Work out the finished part from the listing and answer in its coordinate system (mm). Face numbers are marked on the shaded views. A direction names the side the tool comes from. Coordinates: 2 decimals unless noted, no trailing zeros. Order: outer loops, then holes, each group sorted by start corner. A loop starts at its lowest first (then second) coordinate and runs counter-clockwise, first axis right, second up.
1. The part is cut by section C-C, the plane y = -16. Give the vertices of the cut face in (x, z), then the cut area to 3 significant figures.
2. Flat-ended cylindrical pins translate along their axes: pin 1 Ø4 at (y, z) = (-20.5, 39.5) entering from -X; pin 2 Ø2 at (x, z) = (-16.5, 40.5) entering from -Y; pin 3 Ø5 at (x, y) = (5, -12) entering from +Z; pin 4 Ø2.5 at (x, y) = (6.96, -25.93) entering from -Z. Find the tip coordinate at first contact, or state that the pin passes through.
3. Find the intervals of material crossed by probe 1 along Y at (x, z) = (-11.5, 23); probe 2 along Z at (x, y) = (-24, -26); probe 3 along X at (y, z) = (-19, 27), in increasing order.
4. The part is cut by section A-A, the plane x = -14.5. Give the vertices of the cut face in (y, z).
5. Determine the mould class of the marked faces 6, 7, 8 and 9 for opening direction Z: +Z half, -Z half, draft (parallel to the pull), parting line (faces both ways), or undercut.
6. The part is cut by section D-D, the plane x = -22. Give the vertices of the cut face in (y, z), then the cut area to 3 significant figures.
7. The part is cut by section B-B, the plane z = 50. Give the vertices of the cut face in (x, y), then the cut area to 3 significant figures.
8. A tool of negligible diameter and unlimited length cuts with its end or side. For the marked faces 1, 2, 3, 4 and 5, from which of +Z, -Z, +X, -X, +Y, -Y can it reach the whole face along a straight path? Write none if from no direction.
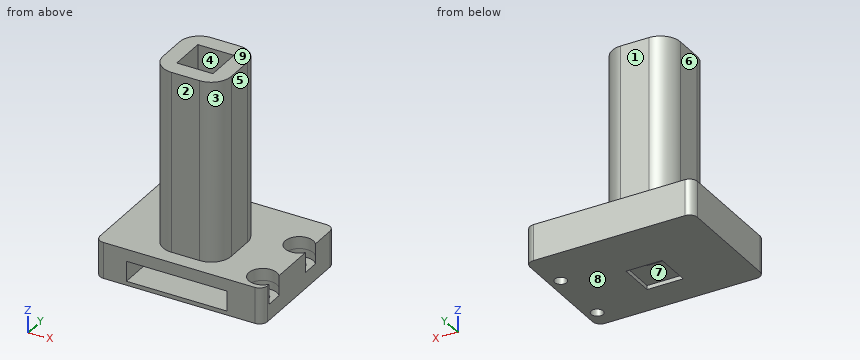
Autodesk Inventor part; units mm, degrees
ref_plane "YZ Plane" through (0, 0, 0) normal (1, 0, 0) x (0, 1, 0)
ref_plane "XZ Plane" through (0, 0, 0) normal (0, 1, 0) x (-1, 0, 0)
ref_plane "XY Plane" through (0, 0, 0) normal (0, 0, 1) x (1, 0, 0)
ref_plane "Work Plane1" through (0, 0, 0) normal (0, 0, 1) x (1, 0, 0)
sketch "Sketch1" plane through (0, 0, 0) normal (0, 0, 1) x (1, 0, 0)
  line L0 (9.7547, 0) -> (-32, 0) construction
  line L1 (-32, 0) -> (-32, -5) construction
  line L2 (-5, -5) -> (-32, -5) construction
  line L3 (-5, -30.7015) -> (-5, -5) construction
  line L4 (-0.2453, -30.7015) -> (-5, -30.7015) construction
  line L5 (-0.2453, -30.7015) -> (-0.2453, -31) construction
  line L6 (-0.2453, -31) -> (4.1607, -31) construction
  line L7 (4.1607, -66) -> (4.1607, -31)
  line L8 (9.7547, -66) -> (4.1607, -66)
  line L9 (9.7547, 0) -> (9.7547, -66)
  circle A0 centre (-2.5, -10.3442) radius 1.45 construction
  circle A1 centre (-2.5, -25.9266) radius 1.45 construction
  circle A2 centre (-11.7453, -18.3978) radius 6 construction
  line L10 (-7.2453, -22.8978) -> (-16.2453, -22.8978)
  line L11 (-16.2453, -22.8978) -> (-16.2453, -13.8978)
  line L12 (-16.2453, -13.8978) -> (-7.2453, -13.8978)
  line L13 (-7.2453, -13.8978) -> (-7.2453, -22.8978)
  line L14 (-7.2453, -22.8978) -> (-16.2453, -13.8978)
  line L15 (-16.2453, -22.8978) -> (-7.2453, -13.8978)
  line L16 (9.7547, 0) -> (-32, 0)
  line L17 (9.7547, 0) -> (-32, 0) construction
  line L18 (-32, 0) -> (-32, -5) construction
  line L19 (-5, -5) -> (-32, -5) construction
  line L20 (-5, -30.7015) -> (-5, -5) construction
  line L21 (-0.2453, -30.7015) -> (-5, -30.7015) construction
  line L22 (-0.2453, -30.7015) -> (-0.2453, -31) construction
  line L23 (-0.2453, -31) -> (4.1607, -31) construction
  line L24 (4.1607, -66) -> (4.1607, -31) construction
  line L25 (9.7547, -66) -> (4.1607, -66) construction
  line L26 (9.7547, 0) -> (9.7547, -66) construction
  circle A3 centre (-2.5, -10.3442) radius 1.45 construction
  circle A4 centre (-2.5, -25.9266) radius 1.45 construction
  line L27 (9.7547, 0) -> (-32, 0)
  line L28 (-32, 0) -> (-32, -30.7015)
  line L29 (-32, -30.7015) -> (9.7547, -30.7015)
  line L30 (9.7547, -30.7015) -> (9.7547, 0)
  circle A5 centre (-2.5, -25.9266) radius 1.65
  circle A6 centre (-2.5, -10.3442) radius 1.65
  circle A7 centre (6.9577, -25.9266) radius 1.45
  circle A8 centre (6.9577, -10.3442) radius 1.45
  circle A9 centre (6.9577, -25.9266) radius 1.45
  circle A10 centre (6.9577, -10.3442) radius 1.45
  point P0 (0, 0)
  dimension "d0" = 9
  dimension "d1" = 9
  dimension "d2" = 3.3
  dimension "d3" = 3.3
extrude "Extrusion1" add sketch "Sketch1" along normal blind 6 contours L9 L29 L28 L16 | A5 | A6 | A7 | A8
sketch "Sketch2" plane through (0, 0, 6) normal (0, 0, 1) x (1, 0, 0)
  circle A0 centre (-2.5, -25.9266) radius 1.65
  circle A1 centre (-2.5, -10.3442) radius 1.65
  circle A2 centre (6.9577, -25.9266) radius 1.45
  circle A3 centre (6.9577, -10.3442) radius 1.45
  point P0 (0, 0)
hole "Hole1" at (6.9577, -25.9266, 6) at (6.9577, -10.3442, 6) direction (0, 0, -1) diameter 3 end through all counterbore diameter 7 counterbore depth 2
fillet "Fillet1" radius 2 4 edges at (-32, 0, 3) (9.7547, 0, 3) (9.7547, -30.7015, 3) (-32, -30.7015, 3)
sketch "Sketch3" plane through (0, 0, 6) normal (0, 0, 1) x (1, 0, 0)
  line L0 (-16.2453, -22.8978) -> (-16.2453, -13.8978)
  line L1 (-7.2453, -13.8978) -> (-7.2453, -22.8978)
  line L2 (-7.2453, -22.8978) -> (-16.2453, -22.8978)
  circle A0 centre (-11.7453, -18.3978) radius 6
  circle A1 centre (-11.7453, -18.3978) radius 12.75
  line L3 (-24.4953, -18.3978) -> (1.0047, -18.3978)
  line L4 (0.7547, -46.1354) -> (-24.2453, -46.1354)
  line L5 (-24.2453, -46.1354) -> (-24.2453, -20.9102)
  line L6 (-24.2453, -20.9102) -> (0.7547, -20.9102)
  line L7 (0.7547, -20.9102) -> (0.7547, -46.1354)
  line L8 (0.7547, -46.1354) -> (-24.2453, -20.9102) construction
  line L9 (-24.2453, -46.1354) -> (0.7547, -20.9102) construction
  point P0 (0, 0)
  point P1 (-11.7453, -33.5228)
  dimension "d14" = 25.5
  dimension "d17" = 25
extrude "Extrusion2" cut sketch "Sketch3" against normal blind 5
sketch "Sketch4" plane through (0, 0, 6) normal (0, 0, 1) x (1, 0, 0)
  line L0 (0.7547, -20.9102) -> (0.7547, -30.7015)
  line L1 (0.7547, -30.7015) -> (7.7547, -30.7015)
  arc A0 (7.7547, -30.7015) -> (9.7547, -28.7015) centre (7.7547, -28.7015) ccw
  line L2 (9.7547, -28.7015) -> (9.7547, -28.0305)
  arc A1 (9.7547, -23.8226) -> (9.7547, -28.0305) centre (6.9577, -25.9266) ccw
  line L3 (9.7547, -23.8226) -> (9.7547, -12.4481)
  arc A2 (9.7547, -8.2402) -> (9.7547, -12.4481) centre (6.9577, -10.3442) ccw
  line L4 (9.7547, -8.2402) -> (9.7547, -2)
  arc A3 (9.7547, -2) -> (7.7547, 0) centre (7.7547, -2) ccw
  line L5 (7.7547, 0) -> (-30, 0)
  arc A4 (-30, 0) -> (-32, -2) centre (-30, -2) ccw
  line L6 (-32, -2) -> (-32, -28.7015)
  arc A5 (-32, -28.7015) -> (-30, -30.7015) centre (-30, -28.7015) ccw
  line L7 (-30, -30.7015) -> (-24.2453, -30.7015)
  line L8 (-24.2453, -30.7015) -> (-24.2453, -20.9102)
  arc A6 (0.7547, -20.9102) -> (-24.2453, -20.9102) centre (-11.7453, -18.3978) ccw
  line L9 (0.7547, -30.7015) -> (7.7547, -30.7015)
  line L10 (-24.2453, -30.7015) -> (0.7547, -30.7015)
  line L11 (-16.2453, -13.8978) -> (-16.2453, -22.8978)
  line L12 (-16.2453, -22.8978) -> (-7.2453, -22.8978)
  line L13 (-7.2453, -13.8978) -> (-16.2453, -13.8978)
  line L14 (-7.2453, -22.8978) -> (-7.2453, -13.8978)
  point P0 (0, 0)
extrude "Extrusion3" add sketch "Sketch4" along normal blind 3
sketch "Sketch5" plane through (0, 0, 9) normal (0, 0, 1) x (1, 0, 0)
  line L0 (-16.2453, -22.8978) -> (-16.2453, -13.8978)
  line L1 (-7.2453, -13.8978) -> (-7.2453, -22.8978)
  line L2 (-7.2453, -22.8978) -> (-16.2453, -22.8978)
  line L3 (-16.2453, -13.8978) -> (-7.2453, -13.8978)
  line L4 (-7.2453, -13.8978) -> (-7.2453, -22.8978)
  line L5 (-7.2453, -22.8978) -> (-16.2453, -22.8978)
  line L6 (-16.2453, -22.8978) -> (-16.2453, -13.8978)
  line L7 (-30, -30.7015) -> (7.7547, -30.7015)
  arc A0 (7.7547, -30.7015) -> (9.7547, -28.7015) centre (7.7547, -28.7015) ccw
  line L8 (9.7547, -28.7015) -> (9.7547, -28.0305)
  arc A1 (9.7547, -23.8226) -> (9.7547, -28.0305) centre (6.9577, -25.9266) ccw
  line L9 (9.7547, -23.8226) -> (9.7547, -12.4481)
  arc A2 (9.7547, -8.2402) -> (9.7547, -12.4481) centre (6.9577, -10.3442) ccw
  line L10 (9.7547, -8.2402) -> (9.7547, -2)
  arc A3 (9.7547, -2) -> (7.7547, 0) centre (7.7547, -2) ccw
  line L11 (7.7547, 0) -> (-30, 0)
  arc A4 (-30, 0) -> (-32, -2) centre (-30, -2) ccw
  line L12 (-32, -2) -> (-32, -28.7015)
  arc A5 (-32, -28.7015) -> (-30, -30.7015) centre (-30, -28.7015) ccw
  line L13 (-3.2453, -9.8978) -> (-20.2453, -9.8978)
  line L14 (-20.2453, -9.8978) -> (-20.2453, -26.8978)
  line L15 (-20.2453, -26.8978) -> (-3.2453, -26.8978)
  line L16 (-3.2453, -26.8978) -> (-3.2453, -9.8978)
  point P0 (0, 0)
  dimension "d20" = 4
extrude "Extrusion4" add sketch "Sketch5" along normal blind 45 contours L16 L15 L14 L13
fillet "Fillet2" radius 5 4 edges at (-3.2453, -26.8978, 31.5) (-20.2453, -26.8978, 31.5) (-3.2453, -9.8978, 31.5) (-20.2453, -9.8978, 31.5)
properties part number "30_cellSTORM_laserbase_ESP32cameradapter_v3"
Geometry says:
1. outline: (-32, 0) - (-16.25, 0) - (-16.25, 1) - (-24.27, 1) - (-24.27, 6) - (-16.25, 6) - (-16.25, 54) - (-20.25, 54) - (-20.25, 9) - (-32, 9) - close; (-7.25, 0) - (9.75, 0) - (9.75, 9) - (-3.25, 9) - (-3.25, 54) - (-7.25, 54) - (-7.25, 6) - (0.78, 6) - (0.78, 1) - (-7.25, 1) - close
1. area: 575 mm2
2. pin 1: stops at x = -20.25
2. pin 2: stops at y = -26.89
2. pin 3: stops at z = 9
2. pin 4: passes through
3. probe 1: y = -26.9 to -22.9, -13.9 to -9.9
3. probe 2: z = 0 to 1, 6 to 9
3. probe 3: x = -20.25 to -16.25, -7.25 to -3.25
4. outline: (-30.7, 0) - (-22.9, 0) - (-22.9, 1) - (-30.7, 1) - close; (-30.7, 6) - (-22.9, 6) - (-22.9, 54) - (-26.9, 54) - (-26.9, 9) - (-30.7, 9) - close; (-13.9, 0) - (0, 0) - (0, 9) - (-9.9, 9) - (-9.9, 54) - (-13.9, 54) - (-13.9, 6) - (-5.95, 6) - (-5.95, 1) - (-13.9, 1) - close
5. face 6: draft
5. face 7: undercut
5. face 8: -Z half
5. face 9: +Z half
6. outline: (-30.7, 0) - (0, 0) - (0, 9) - (-30.7, 9) - (-30.7, 6) - (-10.82, 6) - (-10.82, 1) - (-30.7, 1) - close
6. area: 177 mm2
7. outline: (-20.25, -21.9) arc R5 ccw to (-15.25, -26.9) - (-8.25, -26.9) arc R5 ccw to (-3.25, -21.9) - (-3.25, -14.9) arc R5 ccw to (-8.25, -9.9) - (-15.25, -9.9) arc R5 ccw to (-20.25, -14.9) - close; hole (-16.25, -22.9) - (-7.25, -22.9) - (-7.25, -13.9) - (-16.25, -13.9) - close
7. area: 187 mm2
8. face 1: +Z, +X, -X, +Y
8. face 2: +Z, +X, -X, -Y
8. face 3: +Z, +X, -Y
8. face 4: +Z, -Z
8. face 5: +Z, +X, +Y, -Y
